Geometry: final body of the model. Coordinates: model frame, mm. A direction names the side the tool comes from. Coordinates: 2 decimals unless noted, no trailing zeros. Write each loop counter-clockwise with the first axis right and the second up, starting at its lowest first coordinate (ties: lowest second). Pieces come first, ordered by that corner, then holes.
from build123d import *

# Parameters (mm, degrees)
SKETCH_2_R          = 10
CUT_EXTRUDE_1_DEPTH = 15
CHAMFER_1_SIZE      = 2
FILLET_1_R          = 2
FILLET_2_R          = 10


with BuildPart() as part:
    # 草图1 → 旋转1 (revolve)
    with BuildSketch(Plane.XY, mode=Mode.PRIVATE) as revolve_1_sk:
        Polygon((0, 0), (16, 0), (16, -15), (27.5, -55), (27.5, -80), (0, -80), align=None)
    revolve(revolve_1_sk.sketch.rotate(Axis((0, 36.444043321, 0), (0, -1, 0)), 90), axis=Axis((0, 36.444043321, 0), (0, -1, 0)))

    # 草图2 → 切除-拉伸1 (cut)
    with BuildSketch(Plane(origin=(0, 0, 0), x_dir=(1, 0, 0), z_dir=(0, 1, 0))):
        with Locations(Location((0, 0, 0), (0, 0, 270))):
            Circle(SKETCH_2_R)
    extrude(amount=-CUT_EXTRUDE_1_DEPTH, mode=Mode.SUBTRACT)

    # 倒角1
    chamfer_1_edges = [part.edges().sort_by_distance(p)[0] for p in [
        (0, 0, -10),
    ]]
    chamfer(chamfer_1_edges, length=CHAMFER_1_SIZE)

    # 圆角1
    fillet_1_edges = [part.edges().sort_by_distance(p)[0] for p in [
        (0, -15, -10),
    ]]
    fillet(fillet_1_edges, radius=FILLET_1_R)

    # 圆角2
    fillet_2_edges = [part.edges().sort_by_distance(p)[0] for p in [
        (0, -15, -16),
    ]]
    fillet(fillet_2_edges, radius=FILLET_2_R)


solid = part.part
Item 1: Section A-A, the plane y = -58. Output: boundary loops of the cut face in (x, z).
Derived:
outline: circle Ø55 at (0, 0)
Item 2: Material intervals for probe 1 along X at (y, z) = (-9, 0); probe 2 along Y at (x, z) = (-2.5, -4.5); probe 3 along X at (y, z) = (-61.5, 0), sorted ascending.
Derived:
probe 1: x = -16 to -10, 10 to 16
probe 2: y = -80 to -15
probe 3: x = -27.5 to 27.5
Item 3: Pin query (flat end, axial travel): pin 1 (1.5 mm diameter, centred on x = -3, y = -66.5, fed in from +Z); pin 2 (23 mm diameter, centred on x = 0, z = 0, fed in from +Y); pin 3 (5 mm diameter, centred on y = -47, z = -12, fed in from +X). Return the tip coordinate at first contact, or that it passes through.
Derived:
pin 1: stops at z = 27.41
pin 2: stops at y = -0.5
pin 3: stops at x = 23.6
Item 4: Pull-direction query (Z, two-part tool) for faces 3 (the flat face through (0, -80, 0)), 4 (the cylindrical face through (15.62, -6.89, -3.47)), 5 (the cylindrical face through (-9.76, -7.42, -2.17)); classes: released by +Z, released by -Z, zero draft, split by the parting line, or undercut.
Derived:
face 3: zero draft
face 4: split by the parting line
face 5: undercut
Item 5: Set-up query: faces 1 (the flat face through (0, -15, 0)), 2 (the flat face through (-12, 0, -2)). Return all of +Z, -Z, +X, -X, +Y, -Y with unobstructed straight access to the full face (end or side cutting, diameter ignored); none if empty.
Derived:
face 1: +Y
face 2: +Z, -Z, +X, -X, +Y
